Verification items for this drawing (mm, ordinates from the low corner). A direction names the side the tool comes from. Coordinates: 2 decimals unless noted, no trailing zeros. Order: outer loops, then holes, each group sorted by start corner. A loop starts at its lowest first (then second) coordinate and runs counter-clockwise, first axis right, second up.
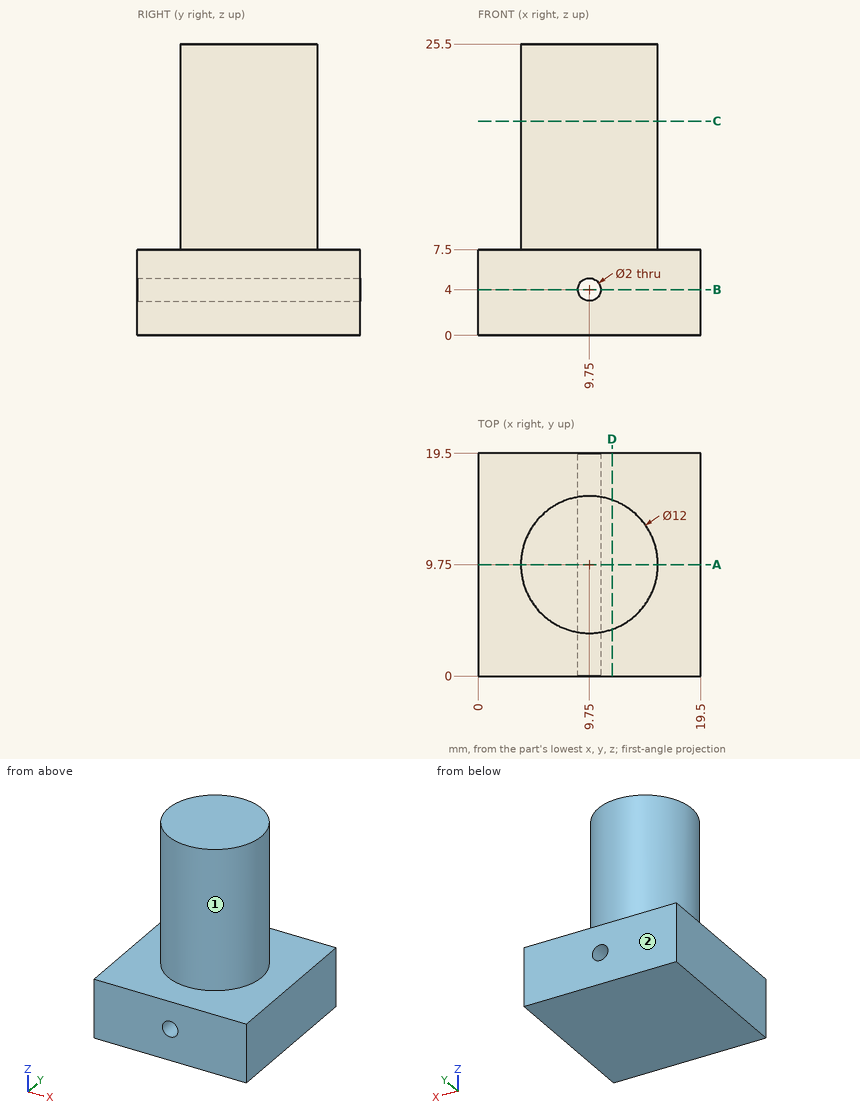
Item 1: Depth check by flat-ended pin: P1, Ø4, axis at y = 6.5, z = 22, coming from the -X side; P2, Ø1.5, axis at x = 4.5, z = 8.5, coming from the -Y side; P3, Ø6, axis at y = 2.5, z = 17.5, coming from the -X side. Enter the tip coordinate at first touch or a pass-through.
Item 2: Sectioned sample at C-C (z = 18.75). Record the cut outline in (x, y).
Item 3: Tool access check on the marked faces 1 and 2. Record the directions out of +Z, -Z, +X, -X, +Y, -Y that give a thin tool (end or side, any length) a straight path to the whole face; none if there is none.
Item 4: Sectioned sample at B-B (z = 4). Record the cut outline in (x, y).
Item 5: Thickness scan on line 1 along Z through (x, y) = (9.75, 15); line 2 along X through (y, z) = (10, 4); line 3 along Z through (x, y) = (5.75, 16). Record the ranges inside material, lowest first.
Item 6: Sectioned sample at A-A (y = 9.75). Record the cut outline in (x, z).
Item 7: Sectioned sample at D-D (x = 11.75). Record the cut outline in (y, z).
Geometry check:
1. P1: stops at x = 3.88
1. P2: stops at y = 5.78
1. P3: stops at x = 5.51
2. outline: circle Ø12 at (9.75, 9.75)
3. face 1: +Z
3. face 2: +Z, -Z, +X, -X, +Y
4. outline: (0, 0) - (8.75, 0) - (8.75, 19.5) - (0, 19.5) - close; (10.75, 0) - (19.5, 0) - (19.5, 19.5) - (10.75, 19.5) - close
5. line 1: z = 0 to 3, 5 to 25.5
5. line 2: x = 0 to 8.75, 10.75 to 19.5
5. line 3: z = 0 to 7.5
6. outline: (0, 0) - (19.5, 0) - (19.5, 7.5) - (15.75, 7.5) - (15.75, 25.5) - (3.75, 25.5) - (3.75, 7.5) - (0, 7.5) - close; hole circle Ø2 at (9.75, 4)
7. outline: (0, 0) - (19.5, 0) - (19.5, 7.5) - (15.41, 7.5) - (15.41, 25.5) - (4.09, 25.5) - (4.09, 7.5) - (0, 7.5) - close
